from build123d import *

# Parameters (mm, degrees)
BOSS_EXTRUDE1_DEPTH = 5.9944
SKETCH2_R           = 5.08
CUT_EXTRUDE1_DEPTH  = 412.816809185
CUT_EXTRUDE2_DEPTH  = 1.27
FILLET1_R           = 6.35


with BuildPart() as part:
    # Sketch1 → Boss-Extrude1 (new body)
    with BuildSketch(Plane(origin=(0, 0, 0), x_dir=(1, 0, 0), z_dir=(0, 1, 0))):
        Polygon((-60.325, 0), (51.435, 0), (198.72934278, -355.6), (-207.61934278, -355.6), align=None)
    extrude(amount=BOSS_EXTRUDE1_DEPTH)

    # Sketch2 → Cut-Extrude1 (cut, through all)
    with BuildSketch(Plane(origin=(0, 5.9944, 0), x_dir=(1, 0, 0), z_dir=(0, 1, 0))):
        with Locations(Location((-4.445, -101.6, 0), (0, 0, 270))):
            Circle(SKETCH2_R)
    extrude(amount=-CUT_EXTRUDE1_DEPTH, mode=Mode.SUBTRACT)

    # Sketch3 → Cut-Extrude2 (cut)
    with BuildSketch(Plane(origin=(0, 5.9944, 0), x_dir=(1, 0, 0), z_dir=(0, 1, 0))):
        with BuildLine():
            add(Edge.make_bspline(
                [(-5.640294118, -118.844607843), (-5.768281461, -118.7980584), (-6.012903349, -118.709088566), (-6.344808892, -118.528644016), (-6.628148212, -118.321295156), (-6.859224633, -118.080893307), (-7.042120778, -117.812676631), (-7.164700527, -117.51094663), (-7.246991297, -117.183653612), (-7.254869453, -116.9546664), (-7.258921569, -116.836887255)],
                knots=[0, 0, 0, 0, 1.173413012, 2.242741344, 3.246972854, 4.190159209, 5.106157181, 6.028734337, 6.986083187, 8, 8, 8, 8], degree=3))
            add(Edge.make_bspline(
                [(-7.258921569, -116.836887255), (-7.256653552, -116.74543812), (-7.252200886, -116.565901343), (-7.213482148, -116.303182669), (-7.152660448, -116.051861575), (-7.060728999, -115.816064709), (-6.94901075, -115.590943888), (-6.806603031, -115.383438523), (-6.644343219, -115.184183893), (-6.45490221, -115.003149717), (-6.246885977, -114.837793075), (-6.022041475, -114.69497982), (-5.7838008, -114.572137861), (-5.531145358, -114.473110122), (-5.264549685, -114.394868468), (-4.984496654, -114.338509959), (-4.689484701, -114.308439202), (-4.488640248, -114.302856801), (-4.385857843, -114.3)],
                knots=[0, 0, 0, 0, 1.020607516, 2.003699488, 2.959093155, 3.90154348, 4.82383827, 5.758924752, 6.705354677, 7.688583181, 8.678343028, 9.668238486, 10.65793052, 11.666964273, 12.693473199, 13.756849753, 14.852065001, 16, 16, 16, 16], degree=3))
            add(Edge.make_bspline(
                [(-4.385857843, -114.3), (-4.204545978, -114.307182695), (-3.846812052, -114.321354376), (-3.325593417, -114.452611845), (-2.831953616, -114.659661213), (-2.448510098, -114.897294215), (-2.168676808, -115.124039422), (-1.984603203, -115.31762303), (-1.82878598, -115.529848563), (-1.699174378, -115.761340468), (-1.604276743, -116.013935686), (-1.53070498, -116.282355633), (-1.491818503, -116.571186294), (-1.485111623, -116.769344483), (-1.481666667, -116.871127451)],
                knots=[0, 0, 0, 0, 1.49991019, 2.959369276, 4.423378123, 5.921390363, 6.678638349, 7.402202754, 8.127755887, 8.854987543, 9.592510724, 10.357767003, 11.156475192, 12, 12, 12, 12], degree=3))
            add(Edge.make_bspline(
                [(-1.481666667, -116.871127451), (-1.485981374, -116.986769655), (-1.494320954, -117.210285987), (-1.572283013, -117.531243569), (-1.696017648, -117.824461788), (-1.875697281, -118.087738493), (-2.102550457, -118.322461305), (-2.37847657, -118.530388471), (-2.705170536, -118.708248837), (-2.946454343, -118.79787135), (-3.072279412, -118.844607843)],
                knots=[0, 0, 0, 0, 1.014624892, 1.96109401, 2.884086684, 3.796937268, 4.744810514, 5.74041467, 6.821667794, 8, 8, 8, 8], degree=3))
            add(Edge.make_bspline(
                [(-3.072279412, -118.844607843), (-2.914859742, -118.900489884), (-2.611977915, -119.008009197), (-2.201301068, -119.233230072), (-1.85753283, -119.508365329), (-1.571190747, -119.822675989), (-1.3501441, -120.184044387), (-1.194321746, -120.588929683), (-1.099246075, -121.036791949), (-1.088702629, -121.349878452), (-1.083235294, -121.512230392)],
                knots=[0, 0, 0, 0, 1.112885226, 2.141236288, 3.106314107, 4.037297253, 4.963019108, 5.91395125, 6.9182732, 8, 8, 8, 8], degree=3))
            add(Edge.make_bspline(
                [(-1.083235294, -121.512230392), (-1.086318941, -121.625474405), (-1.092368202, -121.847627831), (-1.137118864, -122.172750949), (-1.207746531, -122.481606909), (-1.308423274, -122.77502823), (-1.438648283, -123.051876406), (-1.600417225, -123.312302358), (-1.786045911, -123.560068261), (-2.004820521, -123.784957815), (-2.242643145, -123.990398791), (-2.500313239, -124.167920217), (-2.770635203, -124.32272247), (-3.061103925, -124.443446772), (-3.365060773, -124.540441866), (-3.686334259, -124.607785027), (-4.022388276, -124.65413566), (-4.252883136, -124.657501283), (-4.370294118, -124.659215686)],
                knots=[0, 0, 0, 0, 1.064292101, 2.08784667, 3.079199066, 4.038508011, 4.998411814, 5.948603018, 6.916206708, 7.902700801, 8.891891554, 9.865962993, 10.839887915, 11.814545202, 12.81711046, 13.834885875, 14.897119988, 16, 16, 16, 16], degree=3))
            add(Edge.make_bspline(
                [(-4.370294118, -124.659215686), (-4.530450496, -124.655055295), (-4.842398953, -124.646951791), (-5.293729483, -124.565960727), (-5.71503222, -124.441015444), (-6.099384044, -124.257093489), (-6.449092805, -124.034776245), (-6.756260599, -123.768991245), (-7.028635641, -123.471514872), (-7.2545707, -123.134254948), (-7.439104567, -122.764001399), (-7.56324669, -122.360000473), (-7.645470959, -121.927477068), (-7.653310887, -121.628844365), (-7.657352941, -121.474877451)],
                knots=[0, 0, 0, 0, 1.120474225, 2.182430745, 3.200631737, 4.18872885, 5.15617281, 6.094022942, 7.025121698, 7.972298329, 8.92766112, 9.911179284, 10.92306075, 12, 12, 12, 12], degree=3))
            add(Edge.make_bspline(
                [(-7.657352941, -121.474877451), (-7.652474419, -121.306189583), (-7.643139125, -120.983396938), (-7.542148126, -120.525386814), (-7.390372291, -120.11345735), (-7.162821914, -119.754925593), (-6.875293668, -119.443678395), (-6.520899225, -119.188042681), (-6.1048536, -118.982176757), (-5.79972148, -118.891818695), (-5.640294118, -118.844607843)],
                knots=[0, 0, 0, 0, 1.117326705, 2.138060355, 3.0968872, 4.015582046, 4.936209226, 5.891768515, 6.898477863, 8, 8, 8, 8], degree=3))
        make_face()
        with BuildLine():
            add(Edge.make_bspline(
                [(-5.864411765, -116.855563725), (-5.860924518, -116.958010868), (-5.854216871, -117.155065791), (-5.765784417, -117.432384032), (-5.640947106, -117.685224799), (-5.451456684, -117.896691957), (-5.226791082, -118.071851556), (-4.962683383, -118.194777943), (-4.670317297, -118.271397042), (-4.464171965, -118.279918431), (-4.357843137, -118.284313725)],
                knots=[0, 0, 0, 0, 1.049749877, 2.019171811, 2.969415362, 3.930571672, 4.912841927, 5.882263861, 6.9076813, 8, 8, 8, 8], degree=3))
            add(Edge.make_bspline(
                [(-4.357843137, -118.284313725), (-4.267190664, -118.280193467), (-4.087615794, -118.272031584), (-3.823719553, -118.203958648), (-3.574222101, -118.089196592), (-3.337369037, -117.939101774), (-3.129857845, -117.746660089), (-2.978959746, -117.504417071), (-2.889286093, -117.221730721), (-2.880680381, -117.020186607), (-2.876176471, -116.914705882)],
                knots=[0, 0, 0, 0, 0.963702045, 1.909012115, 2.877635224, 3.876069072, 4.883498001, 5.860766905, 6.880404623, 8, 8, 8, 8], degree=3))
            add(Edge.make_bspline(
                [(-2.876176471, -116.914705882), (-2.880320884, -116.806003587), (-2.888257178, -116.597845456), (-2.982975445, -116.307569109), (-3.13119673, -116.055199378), (-3.34173584, -115.85609348), (-3.578520019, -115.695862312), (-3.83314048, -115.57939674), (-4.099621151, -115.506701151), (-4.28164435, -115.49911732), (-4.373406863, -115.495294118)],
                knots=[0, 0, 0, 0, 1.127500904, 2.159094072, 3.142695739, 4.143230944, 5.146793142, 6.108626903, 7.046510837, 8, 8, 8, 8], degree=3))
            add(Edge.make_bspline(
                [(-4.373406863, -115.495294118), (-4.474474554, -115.500065785), (-4.670996862, -115.509344111), (-4.955160717, -115.582421103), (-5.212606095, -115.70863905), (-5.438689503, -115.879739544), (-5.62744998, -116.08395805), (-5.764312365, -116.319650961), (-5.848604785, -116.580214386), (-5.859074542, -116.762592094), (-5.864411765, -116.855563725)],
                knots=[0, 0, 0, 0, 1.078218644, 2.096555407, 3.107271322, 4.119806927, 5.107928669, 6.056056474, 7.009025814, 8, 8, 8, 8], degree=3))
        make_face(mode=Mode.SUBTRACT)
        with BuildLine():
            add(Edge.make_bspline(
                [(-6.262843137, -121.453088235), (-6.261298067, -121.532062003), (-6.258299158, -121.685346403), (-6.227977336, -121.907756099), (-6.187633061, -122.117531737), (-6.120192673, -122.310529782), (-6.039744497, -122.490957051), (-5.938476689, -122.65557316), (-5.82434678, -122.811352176), (-5.641910932, -122.988161746), (-5.395980801, -123.178617287), (-5.069204271, -123.342051313), (-4.722376449, -123.44821201), (-4.482077929, -123.45865686), (-4.360955882, -123.463921569)],
                knots=[0, 0, 0, 0, 0.915735869, 1.777400627, 2.601488155, 3.389611073, 4.143901115, 4.889298653, 5.628545054, 6.377725128, 7.829754517, 9.21892808, 10.59820559, 12, 12, 12, 12], degree=3))
            add(Edge.make_bspline(
                [(-4.360955882, -123.463921569), (-4.244070539, -123.45814149), (-4.011671439, -123.44664916), (-3.673723511, -123.347249825), (-3.351752928, -123.193652736), (-3.104787343, -123.014894989), (-2.92282109, -122.844840257), (-2.804586484, -122.695868496), (-2.699780546, -122.534741789), (-2.62065757, -122.353962845), (-2.552880219, -122.16115171), (-2.512632107, -121.951322958), (-2.482143549, -121.727898463), (-2.479246916, -121.573569079), (-2.477745098, -121.493553922)],
                knots=[0, 0, 0, 0, 1.37269116, 2.72927453, 4.110677498, 5.553914238, 6.296474074, 7.034302579, 7.786136671, 8.550941152, 9.350050124, 10.185625034, 11.059300983, 12, 12, 12, 12], degree=3))
            add(Edge.make_bspline(
                [(-2.477745098, -121.493553922), (-2.483630192, -121.352722772), (-2.495006597, -121.080483782), (-2.60268714, -120.693302545), (-2.770681208, -120.341906837), (-3.013921411, -120.042681729), (-3.300915016, -119.790113634), (-3.635707493, -119.611392315), (-4.00477824, -119.495591574), (-4.264597088, -119.485038711), (-4.398308824, -119.479607843)],
                knots=[0, 0, 0, 0, 1.083575586, 2.094646838, 3.074961835, 4.065731916, 5.047123519, 6.002911055, 6.972229185, 8, 8, 8, 8], degree=3))
            add(Edge.make_bspline(
                [(-4.398308824, -119.479607843), (-4.51307051, -119.48550344), (-4.741293091, -119.497227809), (-5.075791284, -119.595526955), (-5.391477394, -119.758351267), (-5.640183053, -119.936812163), (-5.819703541, -120.111248651), (-5.939709917, -120.259029867), (-6.040242629, -120.422270239), (-6.119512002, -120.601057575), (-6.187716213, -120.79166566), (-6.228262868, -120.999410109), (-6.258258414, -121.220834879), (-6.261284213, -121.374116104), (-6.262843137, -121.453088235)],
                knots=[0, 0, 0, 0, 1.356797633, 2.69821633, 4.088085986, 5.54754192, 6.303274427, 7.045712095, 7.79573256, 8.565314721, 9.357790869, 10.186565194, 11.065698936, 12, 12, 12, 12], degree=3))
        make_face(mode=Mode.SUBTRACT)
    extrude(amount=-CUT_EXTRUDE2_DEPTH, mode=Mode.SUBTRACT)

    # Fillet1
    fillet1_edges = [part.edges().sort_by_distance(p)[0] for p in [
        (198.72934278, 2.9972, 355.6),
        (-207.61934278, 2.9972, 355.6),
        (-60.325, 2.9972, 0),
        (51.435, 2.9972, 0),
    ]]
    fillet(fillet1_edges, radius=FILLET1_R)


solid = part.part
The listing builds one solid part. Answer for the finished solid, in the listing's coordinates (mm). Coordinates: 2 decimals unless noted, no trailing zeros. Loops run counter-clockwise (first coordinate to the right, second up) from the corner with the lowest first, then second, coordinate; pieces in that order, holes last. Notation, with made-up numbers: M 44.5,-36 L 64.5,-36 A9 cw 64.5,-28 Z; hole C 57.5,48.25 d1. An arc over 180 degrees is marked long. Answer in a Markdown table with one row per item.
1) Find section B-B (y = 1). Determine the outline of the cut face in (x, z) (3 decimals), then the cut area to 3 significant figures.
Answers below:
| item | result |
|---|---|
| outline | M -203.983,346.82 L -61.949,3.92 A6.35 ccw -56.082,0 L 47.192,0 A6.35 ccw 53.059,3.92 L 195.093,346.82 A6.35 ccw 189.226,355.6 L -198.116,355.6 A6.35 ccw Z; hole C -4.445,101.6 d10.16 |
| area | 92,000 mm^2 |
2) Given pin 1 (1.5 mm diameter, centred on y = 3.5, z = 308.5, fed in from +X); pin 2 (3 mm diameter, centred on y = 4, z = 100, fed in from -X); pin 3 (6 mm diameter, centred on x = -4.445, z = 101.6, fed in from +Y), each flat-ended and moving along its own axis, determine where each tip first touches the part or whether it passes through.
Answers below:
| item | result |
|---|---|
| pin 1 | x = 179.53 |
| pin 2 | x = -102.37 |
| pin 3 | through |
3) Find section C-C (x = 141.5). Determine the outline of the cut face in (y, z).
Answers below:
| item | result |
|---|---|
| outline | M 0,217.44 L 5.99,217.44 L 5.99,355.6 L 0,355.6 Z |
4) Find section A-A (z = 101.6). Determine the outline of the cut face in (x, y) (3 decimals), then the cut area to 3 significant figures.
Answers below:
| item | result |
|---|---|
| outline | M -102.409,0 L -9.525,0 L -9.525,5.994 L -102.409,5.994 Z; M 0.635,0 L 93.519,0 L 93.519,5.994 L 0.635,5.994 Z |
| area | 1,110 mm^2 |
5) Find section D-D (z = 162.5). Determine the outline of the cut face in (x, y), then the cut area to 3 significant figures.
Answers below:
| item | result |
|---|---|
| outline | M -127.63,0 L 118.74,0 L 118.74,5.99 L -127.63,5.99 Z |
| area | 1,480 mm^2 |
6) Find the intervals of material crossed by probe 1 along X at (y, z) = (2.65, 101.6) (3 decimals); probe 2 along X at (y, z) = (4, 90); probe 3 along Z at (x, y) = (175, 2.6), in increasing order.
Answers below:
| item | result |
|---|---|
| probe 1 | -102.409 to -9.525, 0.635 to 93.519 |
| probe 2 | -97.6 to 88.71 |
| probe 3 | 298.31 to 355.6 |
7) Determine the mould class of faces 1 (the flat face through (123.08, 2.96, 172.97)), 2 (the flat face through (-2, 5.994, 215)), 3 (the cylindrical face through (-2.919, 3.039, 106.445)) for opening direction Z: released by +Z, released by -Z, zero draft, split by the parting line, or undercut.
Answers below:
| item | result |
|---|---|
| face 1 | released by -Z |
| face 2 | zero draft |
| face 3 | undercut |
